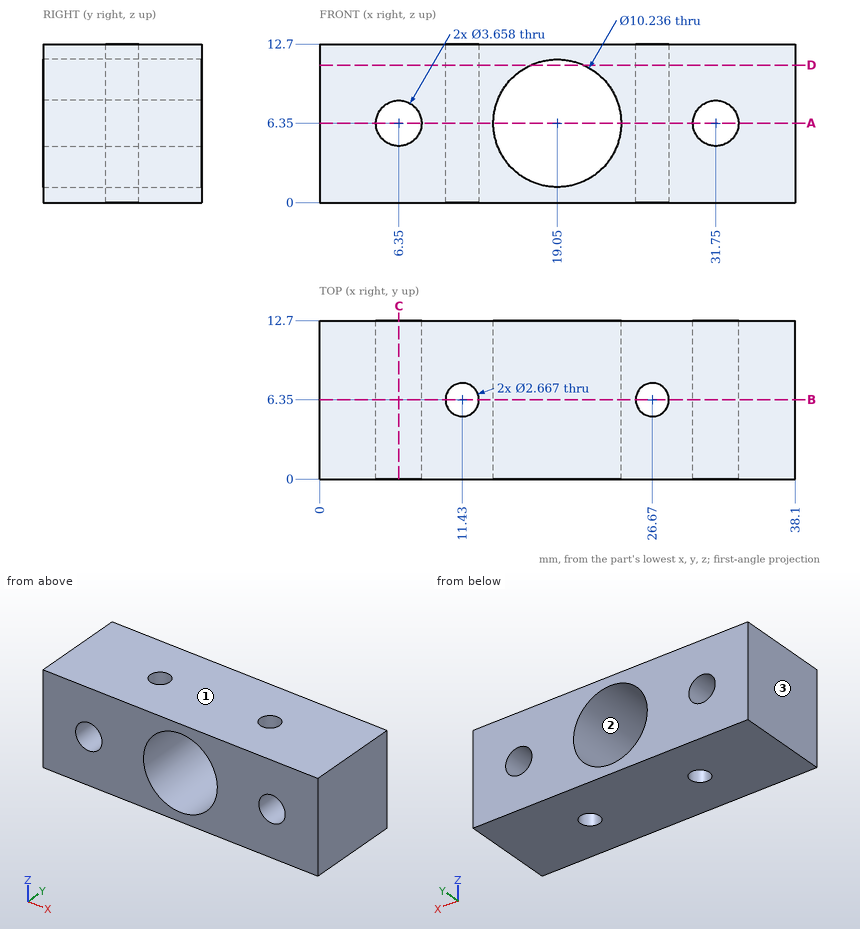
For this review, use the dimensioned drawing (mm, ordinates from the lowest corner) and the shaded views. Round coordinates to 2 decimals unless told otherwise and drop trailing zeros. Write each loop counter-clockwise with the first axis right and the second up, starting at its lowest first coordinate (ties: lowest second). Pieces come first, ordered by that corner, then holes. Notation, with made-up numbers: (50, 83.5) -> (98, 83.5) arc R22 ccw to (98, 106.5) -> close; hole circle Ø8 at (37, 51.25). An arc over 180 degrees is marked (long way). Use CSV: the item, a comma, the result in double quotes.
(1) Draft analysis for pull direction Z (two halves, no side actions). For the marked faces 1, 2 and 3, state which applies: +Z half, -Z half, draft (parallel to the pull), parting line (faces both ways), or undercut.
Computed values:
face 1,"+Z half"
face 2,"undercut"
face 3,"draft"
(2) Consider section D-D, the plane z = 11. Give the boundary of the cut face in (x, y), plus the area to 3 significant figures.
Computed values:
outline,"(0, 0) -> (16.91, 0) -> (16.91, 12.7) -> (0, 12.7) -> close; (21.19, 0) -> (38.1, 0) -> (38.1, 12.7) -> (21.19, 12.7) -> close; hole circle Ø2.67 at (11.43, 6.35); hole circle Ø2.67 at (26.67, 6.35)"
area,"418 mm²"
(3) To check wall thickness, follow L1, parallel to X at y = 6.5, z = 6.35 (1 decimal); L2, parallel to X at y = 3.25, z = 6.35; L3, parallel to Z at x = 33, y = 10 (1 decimal). State the ranges of each line that lie inside material, in increasing order. Write a range as [from, to].
Computed values:
L1,"[0, 4.5], [8.2, 10.1], [12.8, 13.9], [24.2, 25.3], [28, 29.9], [33.6, 38.1]"
L2,"[0, 4.52], [8.18, 13.93], [24.17, 29.92], [33.58, 38.1]"
L3,"[0, 5], [7.7, 12.7]"
(4) Consider section B-B, the plane y = 6.35. Give the boundary of the cut face in (x, z), plus the area to 3 significant figures.
Computed values:
outline,"(0, 0) -> (10.1, 0) -> (10.1, 12.7) -> (0, 12.7) -> close; (12.76, 0) -> (25.34, 0) -> (25.34, 12.7) -> (12.76, 12.7) -> close; (28, 0) -> (38.1, 0) -> (38.1, 12.7) -> (28, 12.7) -> close; hole circle Ø3.66 at (6.35, 6.35); hole circle Ø10.24 at (19.05, 6.35); hole circle Ø3.66 at (31.75, 6.35)"
area,"313 mm²"
(5) Consider section C-C, the plane x = 6.35. Give the boundary of the cut face in (y, z), plus the area to 3 significant figures.
Computed values:
outline,"(0, 0) -> (12.7, 0) -> (12.7, 4.52) -> (0, 4.52) -> close; (0, 8.18) -> (12.7, 8.18) -> (12.7, 12.7) -> (0, 12.7) -> close"
area,"115 mm²"
(6) Consider section A-A, the plane z = 6.35. Give the boundary of the cut face in (x, y).
Computed values:
outline,"(0, 0) -> (4.52, 0) -> (4.52, 12.7) -> (0, 12.7) -> close; (8.18, 0) -> (13.93, 0) -> (13.93, 12.7) -> (8.18, 12.7) -> close; (24.17, 0) -> (29.92, 0) -> (29.92, 12.7) -> (24.17, 12.7) -> close; (33.58, 0) -> (38.1, 0) -> (38.1, 12.7) -> (33.58, 12.7) -> close; hole circle Ø2.67 at (11.43, 6.35); hole circle Ø2.67 at (26.67, 6.35)"
